```python
from build123d import *

# Parameters (mm, degrees)
F0_W      = 90
F0_H      = 74
F1_DEPTH  = 8
F2_W      = 10
F2_H      = 12
F3_DEPTH  = 44
F4_W      = 80
F4_H      = 21
F5_DEPTH  = 25
F6_DEPTH  = 7
F7_W      = 70
F7_H      = 12
F8_DEPTH  = 3
F9_R      = 2
F10_DEPTH = 50
F11_W     = 80
F11_H     = 38
F12_DEPTH = 25
F13_R     = 2
F13_R_2   = 0.7
F14_DEPTH = 25
F15_W     = 5
F15_H     = 35
F16_DEPTH = 5
F17_W     = 5
F17_H     = 35
F18_DEPTH = 20
F20_DEPTH = 50


with BuildPart() as f1:
    # F0 (on Top) → F1 (new body, symmetric)
    with BuildSketch(Plane.XY):
        with Locations((0, 30)):
            Rectangle(F0_W, F0_H)
    extrude(amount=F1_DEPTH, both=True)

    # F2 (on Right) → F3 (cut, symmetric)
    with BuildSketch(Plane.YZ):
        Rectangle(F2_W, F2_H)
    extrude(amount=F3_DEPTH, both=True, mode=Mode.SUBTRACT)

    # F4 (on Top) → F5 (cut)
    with BuildSketch(Plane.XY):
        with Locations((0, 17.5)):
            Rectangle(F4_W, F4_H)
    extrude(amount=F5_DEPTH, mode=Mode.SUBTRACT)

    # F4 (on Top) → F6 (cut)
    with BuildSketch(Plane.XY):
        with Locations((0, 17.5)):
            Rectangle(F4_W, F4_H)
    extrude(amount=-F6_DEPTH, mode=Mode.SUBTRACT)

    # F7 (on face) → F8 (cut)
    with BuildSketch(Plane(origin=(0, 7, 0), x_dir=(-1, 0, 0), z_dir=(0, 1, 0))):
        Rectangle(F7_W, F7_H)
    extrude(amount=-F8_DEPTH, mode=Mode.SUBTRACT)

    # F9 (on Right) → F10 (cut, symmetric)
    with BuildSketch(Plane.YZ):
        Circle(F9_R)
    extrude(amount=F10_DEPTH, both=True, mode=Mode.SUBTRACT)

    # F11 (on face) → F12 (cut)
    with BuildSketch(Plane.XY.offset(8)):
        with Locations((0, 51)):
            Rectangle(F11_W, F11_H)
    extrude(amount=-F12_DEPTH, mode=Mode.SUBTRACT)

    # F13 (on face) → F14 (cut)
    with BuildSketch(Plane.YZ.offset(45)):
        with Locations((51, 0)):
            Circle(F13_R)
        with Locations((44.636039, 6.363961)):
            Circle(F13_R_2)
        with Locations((57.363961, 6.363961)):
            Circle(F13_R_2)
        with Locations((44.636039, -6.363961)):
            Circle(F13_R_2)
        with Locations((57.363961, -6.363961)):
            Circle(F13_R_2)
    extrude(amount=-F14_DEPTH, mode=Mode.SUBTRACT)

    # F15 (on face) → F16 (join)
    with BuildSketch(Plane.XY.offset(8)):
        with Locations((42.5, 49.5)):
            Rectangle(F15_W, F15_H)
        with Locations((-42.5, 49.5)):
            Rectangle(F15_W, F15_H)
    extrude(amount=F16_DEPTH)

    # F17 (on face) → F18 (join)
    with BuildSketch(Plane(origin=(0, 0, -8), x_dir=(1, 0, 0), z_dir=(0, 0, -1))):
        with Locations((42.5, -49.5)):
            Rectangle(F17_W, F17_H)
        with Locations((-42.5, -49.5)):
            Rectangle(F17_W, F17_H)
    extrude(amount=F18_DEPTH)

    # F19 (on Right) → F20 (cut, symmetric)
    with BuildSketch(Plane.YZ):
        with BuildLine():
            Line((56.306477, -10.202515), (64, -16))
            Line((64, -16), (51, -15))
            Line((51, -15), (42.738644, -8))
            Line((42.738644, -8), (30.108895, -8))
            Line((30.108895, -8), (30.108895, -29.582262))
            Line((30.108895, -29.582262), (71.439214, -31.000461))
            Line((71.439214, -31.000461), (73.09068, 17.127901))
            Line((73.09068, 17.127901), (30.442541, 17.835671))
            Line((30.442541, 17.835671), (30.442541, 8))
            Line((30.442541, 8), (42.738644, 8))
            ThreePointArc((42.738644, 8), (60.220396, 6.872721), (56.306477, -10.202515))
        make_face()
    extrude(amount=F20_DEPTH, both=True, mode=Mode.SUBTRACT)


solid = f1.part
```
Here's how the part is built. I have some questions about the finished solid (model axes, mm). A direction names the side the tool comes from. Round coordinates to 2 decimals unless told otherwise and drop trailing zeros. Loops run counter-clockwise (first coordinate to the right, second up) from the corner with the lowest first, then second, coordinate; pieces in that order, holes last. Notation, with made-up numbers: (8, 67.5) -> (20, 67.5) arc R17 ccw to (20, 75.5) -> close; hole circle Ø1 at (70, 23). An arc over 180 degrees is marked (long way). Answer as CSV lines item,"result".
1. Thinking about a two-plate mould opening in Y: for faces 1 (the face through (-1, -7, 0)), 2 (the face through (-45, 28, 1)), 3 (the face through (40, 17, 0)), which applies, released by +Y, released by -Y, zero draft, split by the parting line, or undercut?
Final values:
face 1,"released by -Y"
face 2,"zero draft"
face 3,"undercut"
2. If we section it at B-B on x = -36.5: Please give me the cut outline in (y, z), plus the area to 3 significant figures.
Final values:
outline,"(-7, -8) -> (32, -8) -> (32, 8) -> (28, 8) -> (28, -7) -> (7, -7) -> (7, 8) -> (-7, 8) -> close; hole (-5, -6) -> (5, -6) -> (5, 6) -> (-5, 6) -> close"
area,"189 mm^2"
3. For pin 1 (4 mm diameter, centred on x = -31.5, y = 23, fed in from -Z); pin 2 (1.5 mm diameter, centred on x = 10.5, z = -7.5, fed in from +Y); pin 3 (4.5 mm diameter, centred on y = 51, z = 0, fed in from +X); pin 4 (23 mm diameter, centred on x = -20, y = 20.5, fed in from +Z), each with a flat end and sliding along its axis, tell me the tip position at first contact or that it passes through.
Final values:
pin 1,"stops at z = -8"
pin 2,"stops at y = 32"
pin 3,"stops at x = 45"
pin 4,"stops at z = 8"
4. If we section it at D-D on z = -11.75: Please give me the cut outline in (x, y), plus the area to 3 significant figures.
Final values:
outline,"(-45, 47.16) -> (-40, 47.16) -> (-40, 58.36) -> (-45, 58.36) -> close; (40, 47.16) -> (45, 47.16) -> (45, 58.36) -> (40, 58.36) -> close"
area,"112 mm^2"
5. If I drill on L1, parallel to Z at x = 44.55, y = 0; L2, parallel to Y at x = -6.5, z = 3; L3, parallel to Y at x = 37, z = 6.75, over which ranges is the centre line in solid material (lowest first)?
Final values:
L1,"z = -8 to -2, 2 to 8"
L2,"y = -7 to -5, 28 to 32"
L3,"y = -7 to 7, 28 to 32"
6. Which directions (+Z, -Z, +X, -X, +Y, -Y) give clear straight access to the entire face, cutting with the end or side of a thin tool? Please do faces 4 (the face through (-1, 32, 0)), 5 (the face through (-44, 2.2, 0.1)), 6 (the face through (-1, 28, 0)), 7 (the face through (43, 49, 0)).
Final values:
face 4,"+Z, -Z, +Y"
face 5,"none"
face 6,"+Z"
face 7,"+X"
7. If we section it at C-C on z = 0: Count the separate pieces of the cut face and the enclosed holes in it, plus the area to 3 significant figures.
Final values:
separate pieces,"3"
enclosed holes,"0"
area,"1,090 mm^2"
8. If we section it at A-A on y = 38.5: Please give me the cut outline in (x, z).
Final values:
outline,"(-45, -8) -> (-40, -8) -> (-40, 8) -> (-45, 8) -> close; (40, -8) -> (45, -8) -> (45, 8) -> (40, 8) -> close"
